Could you check a few things on this model? Use its own coordinates, in mm. Round coordinates to 2 decimals unless told otherwise and drop trailing zeros. Write each loop counter-clockwise with the first axis right and the second up, starting at its lowest first coordinate (ties: lowest second). Pieces come first, ordered by that corner, then holes. Notation, with made-up numbers: (43, 59.25) -> (87, 59.25) arc R28 cw to (87, 88.25) -> close; hole circle Ø9 at (-36, 32). An arc over 180 degrees is marked (long way). Return JSON: item names as keys, results as strings.
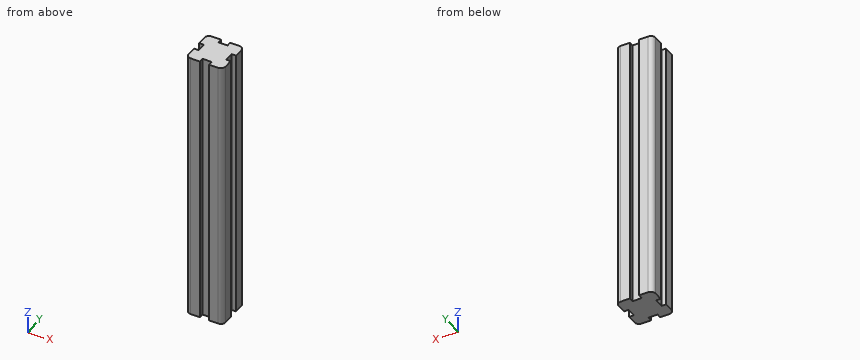
from build123d import *

# Parameters (mm, degrees)
F1_DEPTH = 150
F2_R     = 5


with BuildPart() as f1:
    # F0 (on Top) → F1 (new body, symmetric)
    with BuildSketch(Plane.XY):
        Polygon((20, 5), (20, 20), (5, 20), (5, 15), (-5, 15), (-5, 20), (-20, 20), (-20, 5), (-15, 5), (-15, -5), (-20, -5), (-20, -20), (-5, -20), (-5, -15), (5, -15), (5, -20), (20, -20), (20, -5), (15, -5), (15, 5), align=None)
    extrude(amount=F1_DEPTH, both=True)

    # F2
    f2_edges = [f1.edges().sort_by_distance(p)[0] for p in [
        (20, 20, 0),
        (-20, 20, 0),
        (-20, -20, 0),
        (20, -20, 0),
    ]]
    fillet(f2_edges, radius=F2_R)


solid = f1.part
1) If I drill on probe 1 along Y at (x, z) = (15.5, -17.5); probe 2 along X at (y, z) = (2, 74), over which ranges is the centre line in solid material (lowest first)? Write a range as [from, to].
Return value:
{"probe 1": "[-19.97, -5], [5, 19.97]", "probe 2": "[-15, 15]"}
2) I want a section at B-B, the plane y = 0.5. Please give me the cut outline in (x, z).
Return value:
{"outline": "(-15, -150) -> (15, -150) -> (15, 150) -> (-15, 150) -> close"}
3) Will these pins go through, and if not, where does the flat tip stop? pin 1 Ø2.5 at (x, z) = (-18.5, 74) entering from -Y; pin 2 Ø5 at (x, z) = (1, -55.5) entering from +Y; pin 3 Ø6 at (y, z) = (-2.5, 76.5) entering from -X; pin 4 Ø4 at (y, z) = (-18, -12.5) entering from -X.
Return value:
{"pin 1": "y = -19.47", "pin 2": "y = 15", "pin 3": "x = -20", "pin 4": "x = -19.9"}
4) I want a section at A-A, the plane z = 26. Please give me the cut outline in (x, y).
Return value:
{"outline": "(-20, -15) arc R5 ccw to (-15, -20) -> (-5, -20) -> (-5, -15) -> (5, -15) -> (5, -20) -> (15, -20) arc R5 ccw to (20, -15) -> (20, -5) -> (15, -5) -> (15, 5) -> (20, 5) -> (20, 15) arc R5 ccw to (15, 20) -> (5, 20) -> (5, 15) -> (-5, 15) -> (-5, 20) -> (-15, 20) arc R5 ccw to (-20, 15) -> (-20, 5) -> (-15, 5) -> (-15, -5) -> (-20, -5) -> close"}
